```python
from build123d import *

# Parameters (mm, degrees)
SKETCH1_W           = 3
SKETCH1_H           = 15
SKETCH1_W_2         = 112
SKETCH1_H_2         = 100
SKETCH1_W_3         = 20
SKETCH1_H_3         = 3
BOSS_EXTRUDE1_DEPTH = 3


with BuildPart() as part:
    # Sketch1 → Boss-Extrude1 (new body)
    # profile 1 of 10: a face of its own
    with BuildSketch(Plane.XY):
        with Locations((-57.5, 30)):
            Rectangle(SKETCH1_W, SKETCH1_H)
    # profile 2 of 10: a face of its own
    with BuildSketch(Plane.XY):
        Rectangle(SKETCH1_W_2, SKETCH1_H_2)
        with BuildLine():
            ThreePointArc((-4, 30), (-9, 35), (-14, 30))
            Line((-14, 30), (-14, -30))
            ThreePointArc((-14, -30), (-9, -35), (-4, -30))
            Line((-4, -30), (-4, 30))
        make_face(mode=Mode.SUBTRACT)
        with BuildLine():
            ThreePointArc((-21, 30), (-26, 35), (-31, 30))
            Line((-31, 30), (-31, -30))
            ThreePointArc((-31, -30), (-26, -35), (-21, -30))
            Line((-21, -30), (-21, 30))
        make_face(mode=Mode.SUBTRACT)
        with BuildLine():
            ThreePointArc((-38, 30), (-43, 35), (-48, 30))
            Line((-48, 30), (-48, -30))
            ThreePointArc((-48, -30), (-43, -35), (-38, -30))
            Line((-38, -30), (-38, 30))
        make_face(mode=Mode.SUBTRACT)
        with BuildLine():
            Line((4, -30), (4, 30))
            ThreePointArc((4, 30), (9, 35), (14, 30))
            Line((14, 30), (14, -30))
            ThreePointArc((14, -30), (9, -35), (4, -30))
        make_face(mode=Mode.SUBTRACT)
        with BuildLine():
            Line((21, -30), (21, 30))
            ThreePointArc((21, 30), (26, 35), (31, 30))
            Line((31, 30), (31, -30))
            ThreePointArc((31, -30), (26, -35), (21, -30))
        make_face(mode=Mode.SUBTRACT)
        with BuildLine():
            Line((38, -30), (38, 30))
            ThreePointArc((38, 30), (43, 35), (48, 30))
            Line((48, 30), (48, -30))
            ThreePointArc((48, -30), (43, -35), (38, -30))
        make_face(mode=Mode.SUBTRACT)
    # profile 3 of 10: a face of its own
    with BuildSketch(Plane.XY):
        with Locations((-57.5, 0)):
            Rectangle(SKETCH1_W, SKETCH1_H)
    # profile 4 of 10: a face of its own
    with BuildSketch(Plane.XY):
        with Locations((-35, -51.5)):
            Rectangle(SKETCH1_W_3, SKETCH1_H_3)
    # profile 5 of 10: a face of its own
    with BuildSketch(Plane.XY):
        with Locations((0, -51.5)):
            Rectangle(SKETCH1_W_3, SKETCH1_H_3)
    # profile 6 of 10: a face of its own
    with BuildSketch(Plane.XY):
        with Locations((35, -51.5)):
            Rectangle(SKETCH1_W_3, SKETCH1_H_3)
    # profile 7 of 10: a face of its own
    with BuildSketch(Plane.XY):
        with Locations((57.5, 0)):
            Rectangle(SKETCH1_W, SKETCH1_H)
    # profile 8 of 10: a face of its own
    with BuildSketch(Plane.XY):
        with Locations((57.5, 30)):
            Rectangle(SKETCH1_W, SKETCH1_H)
    # profile 9 of 10: a face of its own
    with BuildSketch(Plane.XY):
        with Locations((-57.5, -30)):
            Rectangle(SKETCH1_W, SKETCH1_H)
    # profile 10 of 10: a face of its own
    with BuildSketch(Plane.XY):
        with Locations((57.5, -30)):
            Rectangle(SKETCH1_W, SKETCH1_H)
    extrude(amount=BOSS_EXTRUDE1_DEPTH)


solid = part.part
```
The model under review builds one solid part; all positions refer to its coordinate system, in mm. A direction names the side the tool comes from. Round coordinates to 2 decimals unless told otherwise and drop trailing zeros. Write each loop counter-clockwise with the first axis right and the second up, starting at its lowest first coordinate (ties: lowest second). Pieces come first, ordered by that corner, then holes. Notation, with made-up numbers: (83.5, -33.75) - (99.5, -33.75) arc R33 ccw to (99.5, 4.25) - close; hole circle Ø1 at (74.25, -16). An arc over 180 degrees is marked (long way). Use one line per item in the form item = value.
Q1. Consider section B-B (x = 23). State the section outline as (y, z) points.
Answer key:
outline = (-50, 0) - (-34, 0) - (-34, 3) - (-50, 3) - close; (34, 0) - (50, 0) - (50, 3) - (34, 3) - close
Q2. Draft analysis for pull direction X (two halves, no side actions). For faces 1 (the flat face through (17, -50, 1)), 2 (the flat face through (45, -52, 1)), 3 (the flat face through (-58, -22.5, 1)), 4 (the flat face through (-48, 0, 1)), state which applies: +X half, -X half, draft (parallel to the pull), parting line (faces both ways), or undercut.
Answer key:
face_1 = undercut
face_2 = +X half
face_3 = draft
face_4 = undercut
Q3. For line 1 (Y direction, x = -26, z = 0.3); line 2 (Y direction, x = 27, z = 1.85); line 3 (X direction, y = 38, z = 1.6), list the stretches that pass through material, from the lowest coordinate up. Write a range as [from, to].
Answer key:
line_1 = [-53, -35], [35, 50]
line_2 = [-53, -34.9], [34.9, 50]
line_3 = [-56, 56]
Q4. Consider section D-D (x = -43). State the section outline as (y, z) points, and give its area (3 significant figures).
Answer key:
outline = (-53, 0) - (-35, 0) - (-35, 3) - (-53, 3) - close; (35, 0) - (50, 0) - (50, 3) - (35, 3) - close
area = 99.0 mm2
Q5. Consider section C-C (y = -18.5). State the section outline as (x, z) points, and give its area (3 significant figures).
Answer key:
outline = (-56, 0) - (-48, 0) - (-48, 3) - (-56, 3) - close; (-38, 0) - (-31, 0) - (-31, 3) - (-38, 3) - close; (-21, 0) - (-14, 0) - (-14, 3) - (-21, 3) - close; (-4, 0) - (4, 0) - (4, 3) - (-4, 3) - close; (14, 0) - (21, 0) - (21, 3) - (14, 3) - close; (31, 0) - (38, 0) - (38, 3) - (31, 3) - close; (48, 0) - (56, 0) - (56, 3) - (48, 3) - close
area = 156 mm2
Q6. Tool access review of faces 5 (the flat face through (-51, -50, 1)), 6 (the flat face through (57, 22.5, 1)), 7 (the flat face through (56, 44, 1)): name each direction out of +Z, -Z, +X, -X, +Y, -Y from which nothing blocks a thin tool from reaching the whole face with its end or side.
Answer key:
face_5 = +Z, -Z, -X, -Y
face_6 = +Z, -Z, +X
face_7 = +Z, -Z, +X, +Y
Q7. Insertion check: pin 1 Ø0.9 at (x, z) = (57.5, 2) entering from -Y; pin 2 Ø0.9 at (y, z) = (16, 2) entering from -X; pin 3 Ø0.9 at (x, z) = (57, 2) entering from +Y. Each pin has a flat end and moves straight along its axis. Give the tip position at first contact, or say it passes through.
Answer key:
pin_1 = -37.5
pin_2 = -56
pin_3 = 37.5
Q8. Consider section A-A (y = -33). State the section outline as (x, z) points, and give its area (3 significant figures).
Answer key:
outline = (-59, 0) - (-47, 0) - (-47, 3) - (-59, 3) - close; (-39, 0) - (-30, 0) - (-30, 3) - (-39, 3) - close; (-22, 0) - (-13, 0) - (-13, 3) - (-22, 3) - close; (-5, 0) - (5, 0) - (5, 3) - (-5, 3) - close; (13, 0) - (22, 0) - (22, 3) - (13, 3) - close; (30, 0) - (39, 0) - (39, 3) - (30, 3) - close; (47, 0) - (59, 0) - (59, 3) - (47, 3) - close
area = 210 mm2
